from build123d import *

# Parameters (mm, degrees)
F0_W     = 50.8
F0_H     = 355.6
F0_R     = 12.7
F1_DEPTH = 6.35
F2_W     = 50.8
F2_H     = 50.8
F3_DEPTH = 6.35


with BuildPart() as f1:
    # F0 (on Top) → F1 (new body)
    with BuildSketch(Plane.XY):
        Rectangle(F0_W, F0_H)
        Circle(F0_R, mode=Mode.SUBTRACT)
    extrude(amount=F1_DEPTH)

    # F2 (on face) → F3 (join)
    with BuildSketch(Plane.XY.offset(6.35)):
        with Locations((0, -152.4)):
            Rectangle(F2_W, F2_H)
        with Locations((0, 152.4)):
            Rectangle(F2_W, F2_H)
    extrude(amount=F3_DEPTH)


solid = f1.part
Model file for the job. Use its own axes, mm. A direction names the side the tool comes from. Coordinates: 2 decimals unless noted, no trailing zeros. Loops run counter-clockwise (first coordinate to the right, second up) from the corner with the lowest first, then second, coordinate; pieces in that order, holes last. Notation, with made-up numbers: (-39.75, -39) -> (-29.75, -39) arc R12 ccw to (-29.75, -16) -> close; hole circle Ø9 at (53.5, -7). An arc over 180 degrees is marked (long way). Use one line per item in the form item = value. Start each with the question number.
(1) Cut at C-C on z = 2. Give the cut face in (x, y).
(2) Tool access for faces 1 (the flat face through (0, 127, 9)), 2 (the flat face through (0, -152, 12.7)): list every direction of +Z, -Z, +X, -X, +Y, -Y with a clear straight run to the whole face (end or side of a thin tool).
(3) Cut at A-A on x = 0. Give the cut face in (y, z), and give its area (3 significant figures).
(4) Cut at B-B on y = 0. Give the cut face in (x, z).
(5) Flat gauge pins, fed straight in: pin 1 (2 mm diameter, centred on y = 43.5, z = 8.5, fed in from -X); pin 2 (2 mm diameter, centred on x = -8.5, y = 18, fed in from +Z). Where does each tip first touch, or does it go through?
(6) Probe probe 1 along Y at (x, z) = (9.5, 11.25); probe 2 along Y at (x, z) = (0, 3.25); probe 3 along X at (y, z) = (1, 4.5). List the from-to ranges inside material, lowest first. Write a range as from..to.
(7) Pull direction Y, two halves, no side cores. Call faces 3 (the flat face through (17, 2, 0)), 4 (the flat face through (0, -177.8, 6)), 5 (the flat face through (17, 2, 6.35)): pulls with the +Y half, pulls with the -Y half, needs draft (parallel to the pull), parting line crosses it, or undercut.
(8) Cut at D-D on y = -88.5. Give the cut face in (x, z).
Values:
q1.outline = (-25.4, -177.8) -> (25.4, -177.8) -> (25.4, 177.8) -> (-25.4, 177.8) -> close; hole circle Ø25.4 at (0, 0)
q2.face_1 = +Z, +X, -X
q2.face_2 = +Z, +X, -X, +Y, -Y
q3.outline = (-177.8, 0) -> (-12.7, 0) -> (-12.7, 6.35) -> (-127, 6.35) -> (-127, 12.7) -> (-177.8, 12.7) -> close; (12.7, 0) -> (177.8, 0) -> (177.8, 12.7) -> (127, 12.7) -> (127, 6.35) -> (12.7, 6.35) -> close
q3.area = 2,740 mm2
q4.outline = (-25.4, 0) -> (-12.7, 0) -> (-12.7, 6.35) -> (-25.4, 6.35) -> close; (12.7, 0) -> (25.4, 0) -> (25.4, 6.35) -> (12.7, 6.35) -> close
q5.pin_1 = through
q5.pin_2 = 6.35
q6.probe_1 = -177.8..-127, 127..177.8
q6.probe_2 = -177.8..-12.7, 12.7..177.8
q6.probe_3 = -25.4..-12.66, 12.66..25.4
q7.face_3 = needs draft
q7.face_4 = pulls with the -Y half
q7.face_5 = undercut
q8.outline = (-25.4, 0) -> (25.4, 0) -> (25.4, 6.35) -> (-25.4, 6.35) -> close
